Verification items for the finished model (mm, model axes). A direction names the side the tool comes from. Give positions to 0.01 mm unless a question says otherwise; leave off trailing zeros. Loops run counter-clockwise (first coordinate to the right, second up) from the corner with the lowest first, then second, coordinate; pieces in that order, holes last. Notation, with made-up numbers: M 45.5,38 L 96.5,38 A17 cw 96.5,50 Z; hole C 70,74 d2. An arc over 180 degrees is marked long. Use a Markdown table: item, result.
from build123d import *

# Parameters (mm, degrees)
SKETCH2_W            = 20
SKETCH2_H            = 40.5
BOSS_EXTRUDE1_DEPTH  = 41
SKETCH3_W            = 20
SKETCH3_H            = 56.4
BOSS_EXTRUDE2_DEPTH  = 2.6
M5_CLEARANCE_HOLE1_D = 5.5


with BuildPart() as part:
    # Sketch2 → Boss-Extrude1 (new body)
    with BuildSketch(Plane(origin=(0, 0, 0), x_dir=(1, 0, 0), z_dir=(0, 1, 0))):
        Rectangle(SKETCH2_W, SKETCH2_H)
    extrude(amount=BOSS_EXTRUDE1_DEPTH)

    # Sketch3 → Boss-Extrude2 (add)
    with BuildSketch(Plane(origin=(0, 28, 0), x_dir=(1, 0, 0), z_dir=(0, 1, 0))):
        Rectangle(SKETCH3_W, SKETCH3_H)
    extrude(amount=BOSS_EXTRUDE2_DEPTH)

    # M5 Clearance Hole1 (through all)
    with Locations(Plane(origin=(0, 30.6, 0), x_dir=(1, 0, 0), z_dir=(0, 1, 0))):
        with Locations((-5, 24), (5, 24), (5, -24), (-5, -24)):
            Hole(M5_CLEARANCE_HOLE1_D / 2)


solid = part.part
(1) Cross-section at A-A on z = 24. Record the cut outline in (x, y).
Results below:
| item | result |
|---|---|
| outline | M -10,28 L -7.75,28 L -7.75,30.6 L -10,30.6 Z; M -2.25,28 L 2.25,28 L 2.25,30.6 L -2.25,30.6 Z; M 7.75,28 L 10,28 L 10,30.6 L 7.75,30.6 Z |
(2) Cross-section at B-B on x = -5. Record the cut outline in (y, z), then the cut area to 3 significant figures.
Results below:
| item | result |
|---|---|
| outline | M 0,-20.25 L 28,-20.25 L 28,-21.25 L 30.6,-21.25 L 30.6,-20.25 L 41,-20.25 L 41,20.25 L 30.6,20.25 L 30.6,21.25 L 28,21.25 L 28,20.25 L 0,20.25 Z; M 28,-28.2 L 30.6,-28.2 L 30.6,-26.75 L 28,-26.75 Z; M 28,26.75 L 30.6,26.75 L 30.6,28.2 L 28,28.2 Z |
| area | 1,670 mm^2 |
(3) Cross-section at C-C on x = -0.75. Record the cut outline in (y, z).
Results below:
| item | result |
|---|---|
| outline | M 0,-20.25 L 28,-20.25 L 28,-28.2 L 30.6,-28.2 L 30.6,-20.25 L 41,-20.25 L 41,20.25 L 30.6,20.25 L 30.6,28.2 L 28,28.2 L 28,20.25 L 0,20.25 Z |
(4) Material ranges on line 1 (Z direction, x = -5, y = 28.7); line 2 (X direction, y = 28.65, z = -24); line 3 (Y direction, x = 0, z = -21.5), recorded low to high.
Results below:
| item | result |
|---|---|
| line 1 | -28.2 to -26.75, -21.25 to 21.25, 26.75 to 28.2 |
| line 2 | -10 to -7.75, -2.25 to 2.25, 7.75 to 10 |
| line 3 | 28 to 30.6 |
(5) Draft check along Z on faces 5 (the flat face through (0, 14, -20.25)), 6 (the flat face through (0, 30.6, -24)), 7 (the cylindrical face through (5.358, 29.282, -26.727)). Enter one of: +Z half, -Z half, draft (parallel to the pull), parting line (faces both ways), or undercut.
Results below:
| item | result |
|---|---|
| face 5 | -Z half |
| face 6 | draft |
| face 7 | undercut |
(6) Set-up check for faces 1 (the flat face through (0, 36, -20.25)), 2 (the flat face through (0, 30.6, 24)), 3 (the flat face through (0, 28, -24)), 4 (the flat face through (0, 14, 20.25)): record each of +Z, -Z, +X, -X, +Y, -Y from which the full face is reachable in a straight line by a thin tool's end or side.
Results below:
| item | result |
|---|---|
| face 1 | -Z, +X, -X, +Y |
| face 2 | +Z, +X, -X, +Y |
| face 3 | -Z, +X, -X, -Y |
| face 4 | +Z, +X, -X, -Y |
(7) Cross-section at D-D on y = 15. Record the cut outline in (x, z).
Results below:
| item | result |
|---|---|
| outline | M -10,-20.25 L 10,-20.25 L 10,20.25 L -10,20.25 Z |
(8) Gauge pin test, flat ends, axial feed: P1, Ø6.5, axis at x = -2.5, z = 25.5, coming from the +Y side; P2, Ø5, axis at x = 0, y = 35, coming from the -Z side; P3, Ø2.5, axis at x = -4.5, z = -23, coming from the +Y side; P4, Ø7, axis at x = 5, z = 24, coming from the -Y side. Record the tip position at first contact, or that the pin passes through.
Results below:
| item | result |
|---|---|
| P1 | y = 30.6 |
| P2 | z = -20.25 |
| P3 | through |
| P4 | y = 28 |
